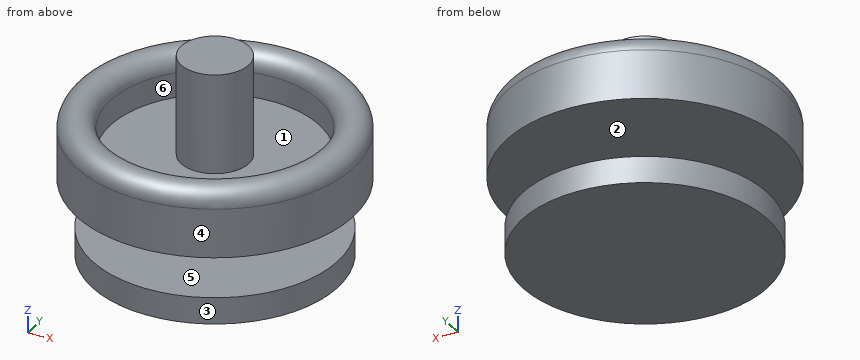
```python
from build123d import *


with BuildPart() as f1:
    # F0 (on Front) → F1 (revolve)
    with BuildSketch(Plane.XZ):
        with BuildLine():
            Line((0, 11), (0, 0))
            Line((0, 0), (50.701149, 0))
            Line((50.701149, 0), (50.701149, 11))
            Line((50.701149, 11), (14, 11))
            Line((14, 11), (14, 31.482756))
            Line((14, 31.482756), (57.156043, 31.482756))
            Line((57.156043, 31.482756), (57.156043, 41.482756))
            Line((57.156043, 41.482756), (57.156043, 51.804224))
            ThreePointArc((57.156043, 51.804224), (50.156043, 59.297508), (43.156043, 51.804224))
            Line((43.156043, 51.804224), (43.156043, 41.482756))
            Line((43.156043, 41.482756), (14, 41.482756))
            Line((14, 41.482756), (14, 51.804224))
            Line((14, 51.804224), (14, 53.735629))
            Line((14, 53.735629), (14, 82.755983))
            Line((14, 82.755983), (0, 82.755983))
            Line((0, 82.755983), (0, 69.811666))
            Line((0, 69.811666), (0, 53.735629))
            Line((0, 53.735629), (0, 11))
        make_face()
    revolve(axis=Axis((0, 0, 32.367814), (0, 0, 1)))


solid = f1.part
```
Could you check a few things on this model? Use its own coordinates, in mm. Face numbers are marked on the shaded views. A direction names the side the tool comes from. Coordinates: 2 decimals unless noted, no trailing zeros. Write each loop counter-clockwise with the first axis right and the second up, starting at its lowest first coordinate (ties: lowest second). Pieces come first, ordered by that corner, then holes. Notation, with made-up numbers: M 39.5,18.25 L 78.5,18.25 A26 ccw 78.5,41.25 Z; hole C 50.5,85.5 d10. An arc over 180 degrees is marked long. Answer as CSV lines item,"result". Start each with the question number.
1) I want a section at D-D, the plane z = 33. Please give me the cut outline in (x, y), and give its area (3 significant figures).
2) I want a section at B-B, the plane y = 0. Please give me the cut outline in (x, z), and give its area (3 significant figures).
3) We'd pull the mould along X, two halves only. Please class the marked faces 4, 5 and 6: +X half, -X half, draft (parallel to the pull), parting line (faces both ways), or undercut.
4) For P1, Ø6, axis at x = 1.5, y = 10, coming from the -Z side; P2, Ø1, axis at y = 5.5, z = 53.5, coming from the -X side; P3, Ø8, axis at y = 33, z = 63.5, coming from the +X side; P4, Ø12, axis at y = 25, z = 36, coming from the +X side, each with a flat end and sliding along its axis, tell me the tip position at first contact or that it passes through.
5) Please list where these lines run through material, in increasing order: line 1 (Y direction, x = 0, z = 49); line 2 (Z direction, x = -20, y = -4); line 3 (Y direction, x = -10, z = 46.5). Write a range as from..to.
6) I want a section at A-A, the plane z = 46.5. Please give me the cut outline in (x, y), and give its area (3 significant figures).
7) For the marked faces 1, 2 and 3, which set-ups out of +Z, -Z, +X, -X, +Y, -Y let a thin tool reach every point of the face, with its end or its side?
Data:
1,outline,"C 0,0 d114.31"
1,area,"10,300 mm^2"
2,outline,"M -57.16,31.48 L -14,31.48 L -14,11 L -50.7,11 L -50.7,0 L 50.7,0 L 50.7,11 L 14,11 L 14,31.48 L 57.16,31.48 L 57.16,51.8 A7.02 ccw long 43.16,51.8 L 43.16,41.48 L 14,41.48 L 14,82.76 L -14,82.76 L -14,41.48 L -43.16,41.48 L -43.16,51.8 A7.02 ccw long -57.16,51.8 Z"
2,area,"4,440 mm^2"
3,face 4,"parting line"
3,face 5,"draft"
3,face 6,"undercut"
4,P1,"stops at z = 0"
4,P2,"stops at x = -56.89"
4,P3,"passes through"
4,P4,"stops at x = 53.91"
5,line 1,"y = -57.16..-43.16, -14..14, 43.16..57.16"
5,line 2,"z = 0..11, 31.48..41.48"
5,line 3,"y = -56.27..-41.98, -9.8..9.8, 41.98..56.27"
6,outline,"C 0,0 d114.31; C 0,0 d28; hole C 0,0 d86.31"
6,area,"5,030 mm^2"
7,face 1,"+Z"
7,face 2,"none"
7,face 3,"-Z"
